CAD build for the part. Positions are in the model's coordinates, mm. Round coordinates to 2 decimals unless told otherwise and drop trailing zeros. Order: outer loops, then holes, each group sorted by start corner. A loop starts at its lowest first (then second) coordinate and runs counter-clockwise, first axis right, second up. Notation, with made-up numbers: (56, 42.5) - (61, 42.5) arc R3 cw to (61, 47.5) - close; hole circle Ø1 at (51, 54). An arc over 180 degrees is marked (long way). Write item = value, one per line.
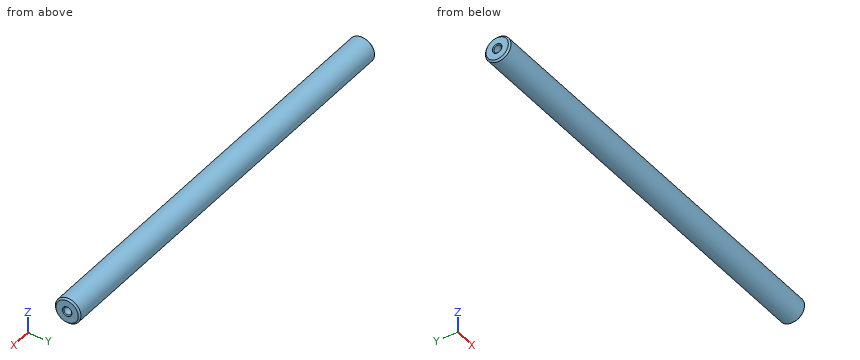
Autodesk Inventor part; units mm, degrees
ref_plane "YZ Plane" through (0, 0, 0) normal (1, 0, 0) x (0, 1, 0)
ref_plane "XZ Plane" through (0, 0, 0) normal (0, 1, 0) x (-1, 0, 0)
ref_plane "XY Plane" through (0, 0, 0) normal (0, 0, 1) x (1, 0, 0)
sketch "Sketch_1" plane through (0, 0, 0) normal (0, 0, 1) x (1, 0, 0)
  line L0 (135, 0) -> (0, 0)
  line L1 (0, 0) -> (0, 3.5)
  line L2 (0, 3.5) -> (0.5, 4)
  line L3 (0.5, 4) -> (134.5, 4)
  line L4 (134.5, 4) -> (135, 3.5)
  line L5 (135, 3.5) -> (135, 0)
  line L6 (135, 0) -> (0, 0)
revolve "Revolution1" add sketch "Sketch_1" angle 360 about axis through (135, 0, 0) along (1, 0, 0)
sketch "Sketch2" plane through (0, 0, 0) normal (-1, 0, 0) x (0, 0, 1)
  point P0 (0, 0)
hole "Hole1" at (0, 0, 0) direction (1, 0, 0) diameter 2.459 depth 8.2901 tip angle 120 countersink diameter 3 countersink angle 90
sketch "Sketch3" plane through (135, 0, 0) normal (1, 0, 0) x (0, 0, -1)
  point P0 (0, 0)
hole "Hole2" at (135, 0, 0) direction (-1, 0, 0) diameter 2.459 depth 8.2901 tip angle 120 countersink diameter 3 countersink angle 90
properties part number "AETTF8-135-M3-N3" material "アルミニウム 2014-T4"
(1) Drop flat-ended pins along their axis: pin 1 (1.5 mm diameter, centred on y = 0, z = 0, fed in from -X); pin 2 (1.5 mm diameter, centred on x = 98.5, y = 1.5, fed in from -Z); pin 3 (3 mm diameter, centred on x = 87, z = -2.5, fed in from -Y). Give the stop position or say it passes through.
Solved:
pin_1 = 8.57
pin_2 = -3.93
pin_3 = -3.87
(2) Band-saw the part on A-A on x = 68. List the corners of the cut face in (y, z).
Solved:
outline = circle Ø8 at (0, 0)
(3) Probe line 1 along Z through (x, y) = (130.75, 0); line 2 along Y through (x, z) = (129, 0.5); line 3 along Z through (x, y) = (108, -1.5). List the from-to ranges inside material, lowest first.
Solved:
line_1 = -4 to -1.23, 1.23 to 4
line_2 = -3.97 to -1.12, 1.12 to 3.97
line_3 = -3.71 to 3.71
